```python
from build123d import *

# Parameters (mm, degrees)
F0_R     = 1.6256
F1_DEPTH = 3.175


with BuildPart() as f1:
    # F0 (on Front) → F1 (new body)
    with BuildSketch(Plane.XZ):
        with BuildLine():
            Line((0, -3.175), (0, 0))
            Line((0, 0), (0, 3.175))
            Line((0, 3.175), (-40.9002420857, 3.175))
            Line((-40.9002420857, 3.175), (-44.45, 3.175))
            Line((-44.45, 3.175), (-44.45, 1.6256))
            ThreePointArc((-44.45, 1.6256), (-43.3005272165, 1.1494727835), (-42.8244, 0))
            ThreePointArc((-42.8244, 0), (-43.3005272165, -1.1494727835), (-44.45, -1.6256))
            Line((-44.45, -1.6256), (-44.45, -3.175))
            Line((-44.45, -3.175), (-40.9002420857, -3.175))
            Line((-40.9002420857, -3.175), (0, -3.175))
        make_face()
        with BuildLine():
            Line((0, 3.175), (0, 0))
            Line((0, 0), (0, -3.175))
            Line((0, -3.175), (40.9002420857, -3.175))
            ThreePointArc((40.9002420857, -3.175), (49.2125, 0), (40.9002420857, 3.175))
            Line((40.9002420857, 3.175), (0, 3.175))
        make_face()
        with BuildLine():
            ThreePointArc((46.0756, 0), (44.45, -1.6256), (42.8244, 0))
            ThreePointArc((42.8244, 0), (44.45, 1.6256), (46.0756, 0))
        make_face(mode=Mode.SUBTRACT)
        with BuildLine():
            ThreePointArc((-47.9997579143, -3.175), (-49.2125, 0), (-47.9997579143, 3.175))
            Line((-47.9997579143, 3.175), (-88.9, 3.175))
            Line((-88.9, 3.175), (-129.8002420857, 3.175))
            ThreePointArc((-129.8002420857, 3.175), (-138.1125, 0), (-129.8002420857, -3.175))
            Line((-129.8002420857, -3.175), (-88.9, -3.175))
            Line((-88.9, -3.175), (-47.9997579143, -3.175))
        make_face()
        with Locations((-133.35, 0)):
            Circle(F0_R, mode=Mode.SUBTRACT)
        with BuildLine():
            Line((-44.45, 1.6256), (-44.45, 3.175))
            Line((-44.45, 3.175), (-47.9997579143, 3.175))
            ThreePointArc((-47.9997579143, 3.175), (-49.2125, 0), (-47.9997579143, -3.175))
            Line((-47.9997579143, -3.175), (-44.45, -3.175))
            Line((-44.45, -3.175), (-44.45, -1.6256))
            ThreePointArc((-44.45, -1.6256), (-46.0756, 0), (-44.45, 1.6256))
        make_face()
        with BuildLine():
            Line((-44.45, -1.6256), (-44.45, 1.6256))
            ThreePointArc((-44.45, 1.6256), (-46.0756, 0), (-44.45, -1.6256))
        make_face()
        with BuildLine():
            ThreePointArc((-42.8244, 0), (-43.3005272165, 1.1494727835), (-44.45, 1.6256))
            Line((-44.45, 1.6256), (-44.45, -1.6256))
            ThreePointArc((-44.45, -1.6256), (-43.3005272165, -1.1494727835), (-42.8244, 0))
        make_face()
    extrude(amount=F1_DEPTH)


solid = f1.part
```
The model under review builds one solid part; all positions refer to its coordinate system, in mm. A direction names the side the tool comes from. Round coordinates to 2 decimals unless told otherwise and drop trailing zeros. Write each loop counter-clockwise with the first axis right and the second up, starting at its lowest first coordinate (ties: lowest second). Pieces come first, ordered by that corner, then holes.
(1) Insertion check: pin 1 (1 mm diameter, centred on x = -4.5, y = -1, fed in from -Z) (3 decimals); pin 2 (1 mm diameter, centred on x = -43.5, y = -1, fed in from +Z) (3 decimals); pin 3 (1 mm diameter, centred on y = -2.5, z = 1, fed in from -X). Each pin has a flat end and moves straight along its axis. Give the tip position at first contact, or say it passes through.
(2) We need section C-C on z = 0. Give the boundary of the cut face in (x, y) (1 decimal).
(3) Machinability: for faces 1 (the flat face through (-43, -2, 3.175)), 2 (the flat face through (-46, -2, -3.175)), 3 (the cylindrical face through (-131.8, -1.57, 0.49)), which of the approach directions +Z, -Z, +X, -X, +Y, -Y give a long, thin tool a straight path to every point of the face, cutting with its end or side? Answer none if there is none.
(4) We need section A-A on x = 44.45. Give the boundary of the cut face in (y, z) (1 decimal).
(5) Wall thickness on L1, parallel to Z at x = -133.35, y = -1.6; L2, parallel to X at y = -0.25, z = 1; L3, parallel to Z at x = -6, y = -2.65 (3 decimals): over which ranges is each line inside the solid? List them lowest first.
(6) Mouldability with a two-part tool opening along X and no side actions: class faces 4 (the flat face through (-46, -3.175, -1)), 5 (the cylindrical face through (-138.11, -1.57, 0.16)) as +X half, -X half, draft (parallel to the pull), parting line (faces both ways), or undercut.
(7) We need section B-B on y = -1.65. Give the number of separate pieces and of enclosed holes in the cut face, and give its area (3 significant figures).
(8) We need section D-D on x = -117.5. Give the boundary of the cut face in (y, z) (3 decimals), and give its area (3 significant figures).
Findings below:
1. pin 1: stops at z = -3.175
1. pin 2: stops at z = 3.175
1. pin 3: stops at x = -138.09
2. outline: (-138.1, -3.2) - (-135, -3.2) - (-135, 0) - (-138.1, 0) - close; (-131.7, -3.2) - (42.8, -3.2) - (42.8, 0) - (-131.7, 0) - close; (46.1, -3.2) - (49.2, -3.2) - (49.2, 0) - (46.1, 0) - close
3. face 1: +Z, +Y, -Y
3. face 2: -Z, +Y, -Y
3. face 3: +Y, -Y
4. outline: (-3.2, -4.8) - (0, -4.8) - (0, -1.6) - (-3.2, -1.6) - close; (-3.2, 1.6) - (0, 1.6) - (0, 4.8) - (-3.2, 4.8) - close
5. L1: z = -4.76 to -1.63, 1.63 to 4.76
5. L2: x = -138.01 to -134.63, -132.07 to 43.17, 45.73 to 49.11
5. L3: z = -3.175 to 3.175
6. face 4: draft
6. face 5: undercut
7. separate pieces: 1
7. enclosed holes: 2
7. area: 1,200 mm2
8. outline: (-3.175, -3.175) - (0, -3.175) - (0, 3.175) - (-3.175, 3.175) - close
8. area: 20.2 mm2
